The listing builds one solid part. Answer for the finished solid, in the listing's coordinates (mm). Round coordinates to 2 decimals unless told otherwise and drop trailing zeros. Loops run counter-clockwise (first coordinate to the right, second up) from the corner with the lowest first, then second, coordinate; pieces in that order, holes last. Notation, with made-up numbers: M 37,-9.5 L 86,-9.5 A20 cw 86,15.5 Z; hole C 60.5,64 d8. An arc over 180 degrees is marked long. Put each result on its own line as item: value. Start each with the question number.
(1) Section A-A, the plane y = -27 is taken. Determine the outline of the cut face in (x, z), then the cut area to 3 significant figures.
(2) Section D-D, the plane y = -9 is taken. Determine the outline of the cut face in (x, z), then the cut area to 3 significant figures.
(3) Flat-ended cylindrical pins translate along their axes: P1, Ø3, axis at y = -9, z = -6, coming from the -X side; P2, Ø10, axis at x = 0.5, y = -24, coming from the +Z side; P3, Ø1, axis at y = -12.5, z = -6, coming from the -X side. Find the tip coordinate at first contact, or state that the pin passes through.
(4) Straight lines are drawn through the part: line 1 (Y direction, x = 4.5, z = -0.5); line 2 (Z direction, x = -7.5, y = -6); line 3 (X direction, y = -15, z = 5.75). For each, find the intervals that lie inside material, in ascending order.
```python
from build123d import *

# Parameters (mm, degrees)
SKETCH1_R           = 8.4963
BOSS_EXTRUDE1_DEPTH = 15.0495
SKETCH3_R           = 0.22225
BOSS_EXTRUDE2_DEPTH = 17.78
SKETCH2_R           = 5.1435
BOSS_EXTRUDE3_DEPTH = 0.000254


with BuildPart() as part:
    # Sketch1 → Boss-Extrude1 (new body)
    with BuildSketch(Plane(origin=(0, 0, 0), x_dir=(1, 0, 0), z_dir=(0, 1, 0))):
        with Locations(Location((0, 0, 0), (0, 0, 270))):
            Circle(SKETCH1_R)
    extrude(amount=-BOSS_EXTRUDE1_DEPTH)

    # Sketch3 → Boss-Extrude2 (add)
    with BuildSketch(Plane(origin=(0, -15.0495, 0), x_dir=(-1, 0, 0), z_dir=(0, -1, 0))):
        with Locations(Location((2.54, 0, 0), (0, 0, 270))):
            Circle(SKETCH3_R)
        with Locations(Location((-2.54, 0, 0), (0, 0, 270))):
            Circle(SKETCH3_R)
    extrude(amount=BOSS_EXTRUDE2_DEPTH)

    # Sketch2 → Boss-Extrude3 (add)
    with BuildSketch(Plane(origin=(0, 0, 0), x_dir=(1, 0, 0), z_dir=(0, 1, 0))):
        with Locations(Location((0, 0, 0), (0, 0, 270))):
            Circle(SKETCH2_R)
    extrude(amount=BOSS_EXTRUDE3_DEPTH)


solid = part.part
```
Recorded:
1. outline: C -2.54,0 d0.44; C 2.54,0 d0.44
1. area: 0.310 mm²
2. outline: C 0,0 d16.99
2. area: 227 mm²
3. P1: stops at x = -7.21
3. P2: stops at z = 0.22
3. P3: stops at x = -6.48
4. line 1: y = -15.05 to 0
4. line 2: z = -3.99 to 3.99
4. line 3: x = -6.25 to 6.25
